Input: part model. Units: mm. Frame: model coordinates. Face numbers are marked on the shaded views. A direction names the side the tool comes from. Give positions to 0.01 mm unless a question says otherwise; leave off trailing zeros. Loops run counter-clockwise (first coordinate to the right, second up) from the corner with the lowest first, then second, coordinate; pieces in that order, holes last. Notation, with made-up numbers: M -33,51 L -18,51 A28 ccw -18,76 Z; hole C 47,82.25 d7. An arc over 180 degrees is marked long. Answer as a JSON object with one key per item and string values. Group by question number.
1) Section query A-A on x = 29.5. Return loops of the section in (y, z) (3 decimals), plus the area to 3 significant figures.
2) First-contact query: P1, Ø1.4, axis at x = -16.51, z = 16.51, coming from the -Y side; P2, Ø1.5, axis at x = -8.5, y = 30.5, coming from the +Z side; P3, Ø5, axis at y = 37, z = -18, coming from the -X side. Flat tips, straight axial feed; report the tip coordinate or a pass-through.
3) Access query for the marked faces 1, 2 and 3. Directions: +Z, -Z, +X, -X, +Y, -Y. A direction counts if a zero-diameter tool reaches every point of the face in a straight line with its end or side. Return the directions, or none.
4) Section query C-C on y = 22. Return loops of the section in (x, z).
5) Section query B-B on z = -5. Return loops of the section in (x, y) (3 decimals), plus the area to 3 significant figures.
6) Draft query along Z for the marked faces 4, 5 and 6. Return one class per face: +Z half, -Z half, draft (parallel to the pull), parting line (faces both ways), or undercut.
7) Section query D-D on x = 10. Return loops of the section in (y, z) (3 decimals).
8) Ray query, L1, parallel to X at y = 36.25, z = -16.51; L2, parallel to X at y = 39.5, z = 17.5. Return the intervals inside material, ascending.
from build123d import *

# Parameters (mm, degrees)
SKETCH1_W                 = 76.2
SKETCH1_H                 = 76.2
EXTRUDE1_DEPTH            = 9.525
SKETCH2_W                 = 68.58
SKETCH2_H                 = 68.58
EXTRUDE2_DEPTH            = 0.79375
SKETCH6_W                 = 50.8
SKETCH6_H                 = 50.8
EXTRUDE4_DEPTH            = 36.195
F_4_40_TAPPED_HOLE1_D     = 2.2606
F_4_40_TAPPED_HOLE1_DEPTH = 12.7
F_4_40_TAPPED_HOLE1_TIP   = 0.679152758
FILLET1_R                 = 0.254


with BuildPart() as part:
    # Sketch1 → Extrude1 (new body)
    with BuildSketch(Plane(origin=(0, 0, 0), x_dir=(1, 0, 0), z_dir=(0, 1, 0))):
        Rectangle(SKETCH1_W, SKETCH1_H)
    extrude(amount=EXTRUDE1_DEPTH)

    # Sketch2 → Extrude2 (cut)
    with BuildSketch(Plane.XZ):
        Rectangle(SKETCH2_W, SKETCH2_H)
    extrude(amount=-EXTRUDE2_DEPTH, mode=Mode.SUBTRACT)

    # Sketch6 → Extrude4 (add)
    with BuildSketch(Plane(origin=(0, 9.525, 0), x_dir=(1, 0, 0), z_dir=(0, 1, 0))):
        Rectangle(SKETCH6_W, SKETCH6_H)
    extrude(amount=EXTRUDE4_DEPTH)

    # #4-40 Tapped Hole1
    with Locations(Plane(origin=(-16.51, 45.72, -16.51), x_dir=(0, 0, 1), z_dir=(0, 1, 0))):
        with Locations((0, 0), (33.02, 0), (33.02, 33.02), (0, 33.02)):
            Hole(F_4_40_TAPPED_HOLE1_D / 2, depth=F_4_40_TAPPED_HOLE1_DEPTH)
            with Locations((0, 0, -(F_4_40_TAPPED_HOLE1_DEPTH + F_4_40_TAPPED_HOLE1_TIP / 2))):  # 118° drill point
                Cone(0, F_4_40_TAPPED_HOLE1_D / 2, F_4_40_TAPPED_HOLE1_TIP, mode=Mode.SUBTRACT)

    # Fillet1
    fillet1_edges = [part.edges().sort_by_distance(p)[0] for p in [
        (16.51, 45.72, -15.3797),
        (16.51, 45.72, 17.6403),
        (-16.51, 45.72, 17.6403),
        (-16.51, 45.72, -15.3797),
    ]]
    fillet(fillet1_edges, radius=FILLET1_R)


solid = part.part
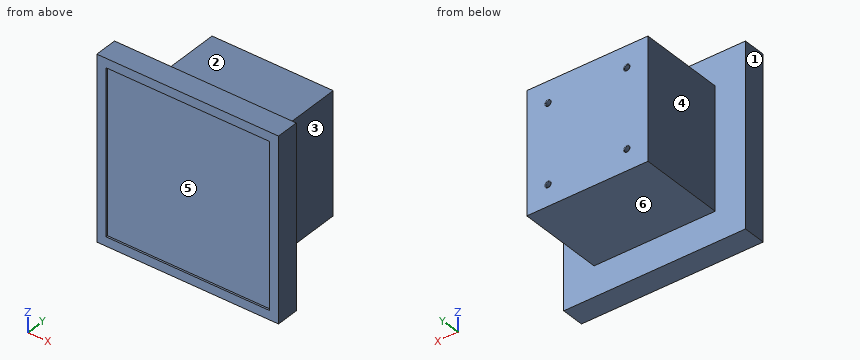
Output:
{
 "1": {"outline": "M 0,-38.1 L 9.525,-38.1 L 9.525,38.1 L 0,38.1 L 0,34.29 L 0.794,34.29 L 0.794,-34.29 L 0,-34.29 Z", "area": "671 mm^2"},
 "2": {"P1": "stops at y = 0.79", "P2": "stops at z = 25.4", "P3": "stops at x = -25.4"},
 "3": {"face 1": "+Z, -Z, -X, +Y, -Y", "face 2": "+Z, +X, -X, +Y", "face 3": "+Z, -Z, +X, +Y"},
 "4": {"outline": "M -25.4,-25.4 L 25.4,-25.4 L 25.4,25.4 L -25.4,25.4 Z"},
 "5": {"outline": "M -38.1,0 L -34.29,0 L -34.29,0.794 L 34.29,0.794 L 34.29,0 L 38.1,0 L 38.1,9.525 L 25.4,9.525 L 25.4,45.72 L -25.4,45.72 L -25.4,9.525 L -38.1,9.525 Z", "area": "2,510 mm^2"},
 "6": {"face 4": "draft", "face 5": "undercut", "face 6": "-Z half"},
 "7": {"outline": "M 0,-38.1 L 9.525,-38.1 L 9.525,-25.4 L 45.72,-25.4 L 45.72,25.4 L 9.525,25.4 L 9.525,38.1 L 0,38.1 L 0,34.29 L 0.794,34.29 L 0.794,-34.29 L 0,-34.29 Z"},
 "8": {"L1": "x = -25.4 to -17.64, -15.38 to 15.38, 17.64 to 25.4", "L2": "x = -25.4 to -17.06, -15.96 to 15.96, 17.06 to 25.4"}
}
